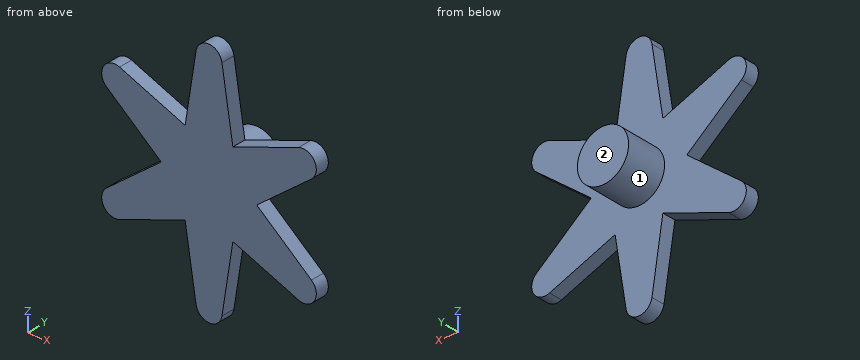
from build123d import *

# Parameters (mm, degrees)
SKETCH1_R           = 7
BOSS_EXTRUDE1_DEPTH = 2
BOSS_EXTRUDE2_START = -2
BOSS_EXTRUDE2_DEPTH = 2
CIRPATTERN1_COUNT   = 6
SKETCH3_R           = 3.75
BOSS_EXTRUDE3_DEPTH = 6


with BuildPart() as part:
    # Sketch1 → Boss-Extrude1 (new body)
    with BuildSketch(Plane(origin=(0, 0, 0), x_dir=(1, 0, 0), z_dir=(0, 1, 0))):
        with Locations(Location((0, 0, 0), (0, 0, 270))):
            Circle(SKETCH1_R)
    extrude(amount=BOSS_EXTRUDE1_DEPTH)

    # Sketch2 → Boss-Extrude2 (add)
    with BuildSketch(Plane(origin=(0, 2, 0), x_dir=(1, 0, 0), z_dir=(0, 1, 0)).offset(BOSS_EXTRUDE2_START)):
        with BuildLine():
            Line((-3.5, 6.062177826), (-1.9, 16.23236311))
            ThreePointArc((-1.9, 16.23236311), (0, 17.856819334), (1.9, 16.23236311))
            Line((1.9, 16.23236311), (3.5, 6.062177826))
            ThreePointArc((3.5, 6.062177826), (0, 7), (-3.5, 6.062177826))
        make_face()
    boss_extrude2 = extrude(amount=BOSS_EXTRUDE2_DEPTH)

    # CirPattern1: Boss-Extrude2 ×6 about axis
    cirpattern1_axis = Axis((0, 0, 0), (0, 1, 0))
    for i in range(1, CIRPATTERN1_COUNT):
        add(boss_extrude2.rotate(cirpattern1_axis, i * 360 / CIRPATTERN1_COUNT))

    # Sketch3 → Boss-Extrude3 (add)
    with BuildSketch(Plane(origin=(0, 2, 0), x_dir=(1, 0, 0), z_dir=(0, 1, 0))):
        with Locations(Location((0, 0, 0), (0, 0, 270))):
            Circle(SKETCH3_R)
    extrude(amount=BOSS_EXTRUDE3_DEPTH)


solid = part.part
Geometry check sheet. Reference: the model listing, model coordinates, mm. Face numbers are marked on the shaded views. A direction names the side the tool comes from. Coordinates: 2 decimals unless noted, no trailing zeros. Order: outer loops, then holes, each group sorted by start corner. A loop starts at its lowest first (then second) coordinate and runs counter-clockwise, first axis right, second up. Notation, with made-up numbers: (-39.75, 19.25) - (-2.75, 19.25) arc R6 cw to (-2.75, 25.25) - close; hole circle Ø11 at (74, 62.25). An arc over 180 degrees is marked (long way). Answer in a Markdown table with one row per item. Add a question column.
1) Cross-section at D-D, the plane x = 0. Record the cut outline in (y, z), then the cut area to 3 significant figures.
2) Material ranges on line 1 along Y through (x, z) = (6.5, -0.5); line 2 along Z through (x, y) = (-8.5, 0.5); line 3 along X through (y, z) = (5, -0.5), recorded low to high. Write a range as [from, to].
3) Cross-section at C-C, the plane x = 10. Record the cut outline in (y, z).
4) Gauge pin test, flat ends, axial feed: P1, Ø2, axis at x = 2, z = 5.5, coming from the +Y side; P2, Ø4, axis at y = 4.5, z = 9.5, coming from the +X side; P3, Ø1.5, axis at y = 4.5, z = -3.5, coming from the +X side. Record the tip position at first contact, or that the pin passes through.
5) Cross-section at A-A, the plane z = 8. Record the cut outline in (x, y).
6) Cross-section at B-B, the plane y = 1.5. Record the cut outline in (x, z), then the cut area to 3 significant figures.
7) Set-up check for the marked faces 1 and 2: record each of +Z, -Z, +X, -X, +Y, -Y from which the full face is reachable in a straight line by a thin tool's end or side.
Check result:
| question | item | result |
|---|---|---|
| 1 | outline | (0, -17.86) - (2, -17.86) - (2, -3.75) - (8, -3.75) - (8, 3.75) - (2, 3.75) - (2, 17.86) - (0, 17.86) - close |
| 1 | area | 116 mm² |
| 2 | line 1 | y = [0, 2] |
| 2 | line 2 | z = [-7.99, -1.21], [1.21, 7.99] |
| 2 | line 3 | x = [-3.72, 3.72] |
| 3 | outline | (0, -8.57) - (2, -8.57) - (2, -2.42) - (0, -2.42) - close; (0, 2.42) - (2, 2.42) - (2, 8.57) - (0, 8.57) - close |
| 4 | P1 | stops at y = 2 |
| 4 | P2 | passes through |
| 4 | P3 | stops at x = 2.55 |
| 5 | outline | (-15.72, 0) - (-8.53, 0) - (-8.53, 2) - (-15.72, 2) - close; (-3.2, 0) - (3.2, 0) - (3.2, 2) - (-3.2, 2) - close; (8.53, 0) - (15.72, 0) - (15.72, 2) - (8.53, 2) - close |
| 6 | outline | (-15.01, -6.47) arc R1.92 ccw to (-13.11, -9.76) - (-3.5, -6.06) - (-1.9, -16.23) arc R1.92 ccw to (1.9, -16.23) - (3.5, -6.06) - (13.11, -9.76) arc R1.92 ccw to (15.01, -6.47) - (7, 0) - (15.01, 6.47) arc R1.92 ccw to (13.11, 9.76) - (3.5, 6.06) - (1.9, 16.23) arc R1.92 ccw to (-1.9, 16.23) - (-3.5, 6.06) - (-13.11, 9.76) arc R1.92 ccw to (-15.01, 6.47) - (-7, 0) - close |
| 6 | area | 485 mm² |
| 7 | face 1 | +Y |
| 7 | face 2 | +Z, -Z, +X, -X, +Y |
